Part model, mm, in its own coordinate system. Coordinates: 2 decimals unless noted, no trailing zeros. Write each loop counter-clockwise with the first axis right and the second up, starting at its lowest first coordinate (ties: lowest second). Pieces come first, ordered by that corner, then holes. Notation, with made-up numbers: (38, 35) - (56, 35) arc R23 ccw to (56, 66) - close; hole circle Ø4 at (-26.5, -16). An arc over 180 degrees is marked (long way). Write each question's results on one line, items separated by ' | '.
from build123d import *

# Parameters (mm, degrees)
BOSS_EXTRUDE1_START = 71.584968
BOSS_EXTRUDE1_DEPTH = 2.5
BOSS_EXTRUDE2_DEPTH = 2.5


with BuildPart() as part:
    # Sketch2 → Boss-Extrude1 (new body)
    with BuildSketch(Plane.XY.offset(-64.584967839).offset(BOSS_EXTRUDE1_START)):
        with BuildLine():
            Line((144.480934022, 643.250628573), (197.480934022, 643.250628573))
            ThreePointArc((197.480934022, 643.250628573), (210.562409474, 648.669153121), (215.980934022, 661.750628573))
            Line((215.980934022, 661.750628573), (215.980934022, 693.750628573))
            ThreePointArc((215.980934022, 693.750628573), (210.562409474, 706.832104025), (197.480934022, 712.250628573))
            Line((197.480934022, 712.250628573), (144.480934022, 712.250628573))
            ThreePointArc((144.480934022, 712.250628573), (131.39945857, 706.832104025), (125.980934022, 693.750628573))
            Line((125.980934022, 693.750628573), (125.980934022, 661.750628573))
            ThreePointArc((125.980934022, 661.750628573), (131.39945857, 648.669153121), (144.480934022, 643.250628573))
        make_face()
        with BuildLine():
            Line((144.480934022, 644.750628573), (197.480934022, 644.750628573))
            ThreePointArc((197.480934022, 644.750628573), (209.501749302, 649.729813293), (214.480934022, 661.750628573))
            Line((214.480934022, 661.750628573), (214.480934022, 693.750628573))
            ThreePointArc((214.480934022, 693.750628573), (209.501749302, 705.771443853), (197.480934022, 710.750628573))
            Line((197.480934022, 710.750628573), (144.480934022, 710.750628573))
            ThreePointArc((144.480934022, 710.750628573), (132.460118742, 705.771443853), (127.480934022, 693.750628573))
            Line((127.480934022, 693.750628573), (127.480934022, 661.750628573))
            ThreePointArc((127.480934022, 661.750628573), (132.460118742, 649.729813293), (144.480934022, 644.750628573))
        make_face(mode=Mode.SUBTRACT)
    extrude(amount=BOSS_EXTRUDE1_DEPTH)

    # Sketch3 → Boss-Extrude2 (add)
    with BuildSketch(Plane.XY.offset(7)):
        with BuildLine():
            Line((125.980934022, 693.750628573), (125.980934022, 661.750628573))
            ThreePointArc((125.980934022, 661.750628573), (131.39945857, 648.669153121), (144.480934022, 643.250628573))
            Line((144.480934022, 643.250628573), (197.480934022, 643.250628573))
            ThreePointArc((197.480934022, 643.250628573), (210.562409474, 648.669153121), (215.980934022, 661.750628573))
            Line((215.980934022, 661.750628573), (215.980934022, 693.750628573))
            ThreePointArc((215.980934022, 693.750628573), (210.562409474, 706.832104025), (197.480934022, 712.250628573))
            Line((197.480934022, 712.250628573), (144.480934022, 712.250628573))
            ThreePointArc((144.480934022, 712.250628573), (131.39945857, 706.832104025), (125.980934022, 693.750628573))
        make_face()
    extrude(amount=BOSS_EXTRUDE2_DEPTH)


solid = part.part
(1) Saw through at A-A on x = 136.5. Write the cut outline in (y, z), then the cut area to 3 significant figures.
Return value:
outline: (645.06, 7) - (710.44, 7) - (710.44, 9.5) - (645.06, 9.5) - close | area: 163 mm^2
(2) Saw through at B-B on z = 8.95. Write the cut outline in (x, y).
Return value:
outline: (125.98, 661.75) arc R18.5 ccw to (144.48, 643.25) - (197.48, 643.25) arc R18.5 ccw to (215.98, 661.75) - (215.98, 693.75) arc R18.5 ccw to (197.48, 712.25) - (144.48, 712.25) arc R18.5 ccw to (125.98, 693.75) - close
(3) Wall check: line 1 (X direction, y = 695, z = 8.35); line 2 (X direction, y = 704.5, z = 8.4); line 3 (Y direction, x = 134, z = 7.2). Give the ranges that are in metal, low to high. Write a range as from..to.
Return value:
line 1: x = 126.02..215.94 | line 2: x = 129.42..212.54 | line 3: y = 646.51..709
